Can you work these out from the model? Positions are in its coordinate system, mm. A direction names the side the tool comes from. Give positions to 0.01 mm unless a question says otherwise; leave off trailing zeros. Write each loop counter-clockwise with the first axis right and the second up, starting at its lowest first coordinate (ties: lowest second). Pieces come first, ordered by that corner, then holes. Notation, with made-up numbers: (28.25, 74.5) -> (44.25, 74.5) arc R28 ccw to (44.25, 93.5) -> close; hole circle Ø8 at (36.25, 29.25). An arc over 180 degrees is marked (long way). One line per item, written item: value.
from build123d import *

# Parameters (mm, degrees)
F0_W     = 65
F0_H     = 25
F1_DEPTH = 2
F2_W     = 3
F2_H     = 25
F3_DEPTH = 66
F4_R     = 4
F4_R_2   = 1.5
F5_DEPTH = 65.001


with BuildPart() as f1:
    # F0 (on Top) → F1 (new body)
    with BuildSketch(Plane.XY):
        with Locations((32.5, 12.5)):
            Rectangle(F0_W, F0_H)
    extrude(amount=F1_DEPTH)

    # F2 (on Top) → F3 (join)
    with BuildSketch(Plane.XY):
        with Locations((1.5, 12.5)):
            Rectangle(F2_W, F2_H)
        with Locations((63.5, 12.5)):
            Rectangle(F2_W, F2_H)
    extrude(amount=F3_DEPTH)

    # F4 (on face) → F5 (cut, through all)
    with BuildSketch(Plane(origin=(0, 0, 0), x_dir=(0, -1, 0), z_dir=(-1, 0, 0))):
        with BuildLine():
            ThreePointArc((-25, 53.5), (-21.338835, 62.338835), (-12.5, 66))
            Line((-12.5, 66), (-25, 66))
            Line((-25, 66), (-25, 53.5))
        make_face()
        with BuildLine():
            ThreePointArc((-12.5, 66), (-3.661165, 62.338835), (0, 53.5))
            Line((0, 53.5), (0, 66))
            Line((0, 66), (-12.5, 66))
        make_face()
        with Locations((-12.5, 53.5)):
            Circle(F4_R)
        with Locations((-12.5, 60.5)):
            Circle(F4_R_2)
        with Locations((-19.5, 53.5)):
            Circle(F4_R_2)
        with Locations((-12.5, 46.5)):
            Circle(F4_R_2)
        with Locations((-5.5, 53.5)):
            Circle(F4_R_2)
    extrude(amount=-F5_DEPTH, mode=Mode.SUBTRACT)


solid = f1.part
1) Will this pin go through, and if not, where does the flat tip stop? pin 1 (1.5 mm diameter, centred on x = 24.5, y = 5.5, fed in from +Z).
Answer list:
pin 1: stops at z = 2
2) If we section it at C-C (z = 60.5): Write out the boundary of the cut face in (x, y).
Answer list:
outline: (0, 2.14) -> (3, 2.14) -> (3, 11) -> (0, 11) -> close; (0, 14) -> (3, 14) -> (3, 22.86) -> (0, 22.86) -> close; (62, 2.14) -> (65, 2.14) -> (65, 11) -> (62, 11) -> close; (62, 14) -> (65, 14) -> (65, 22.86) -> (62, 22.86) -> close
3) I need wall thicknesses on L1, parallel to Z at x = 63.25, y = 12.5; L2, parallel to X at y = 20.75, z = 54.5; L3, parallel to Z at x = 0.9, y = 19.5. Which ranges of each line are inside material? Lowest first, please.
Answer list:
L1: z = 0 to 45, 48 to 49.5, 57.5 to 59, 62 to 66
L2: x = 0 to 3, 62 to 65
L3: z = 0 to 52, 55 to 63.86
4) If we section it at A-A (z = 9.5): Write out the boundary of the cut face in (x, y), and give its area (3 significant figures).
Answer list:
outline: (0, 0) -> (3, 0) -> (3, 25) -> (0, 25) -> close; (62, 0) -> (65, 0) -> (65, 25) -> (62, 25) -> close
area: 150 mm^2
5) We'd pull the mould along X, two halves only. Please class faces 3 (the face through (3, 12, 34)), 4 (the face through (65, 12, 33)), 5 (the face through (1.479, 12.695, 61.987)): released by +X, released by -X, zero draft, split by the parting line, or undercut.
Answer list:
face 3: undercut
face 4: released by +X
face 5: zero draft
6) For faces 1 (the face through (62, 12, 34)), 2 (the face through (1.479, 13.367, 49.595)), which set-ups out of +Z, -Z, +X, -X, +Y, -Y let a thin tool reach every point of the face, with its end or its side?
Answer list:
face 1: +Z, +Y, -Y
face 2: +X, -X
7) If we section it at D-D (y = 2): Write out the boundary of the cut face in (x, z).
Answer list:
outline: (0, 0) -> (65, 0) -> (65, 60.28) -> (62, 60.28) -> (62, 2) -> (3, 2) -> (3, 60.28) -> (0, 60.28) -> close
8) If we section it at B-B (y = 19.5): Write out the boundary of the cut face in (x, z), and give its area (3 significant figures).
Answer list:
outline: (0, 0) -> (65, 0) -> (65, 52) -> (62, 52) -> (62, 2) -> (3, 2) -> (3, 52) -> (0, 52) -> close; (0, 55) -> (3, 55) -> (3, 63.86) -> (0, 63.86) -> close; (62, 55) -> (65, 55) -> (65, 63.86) -> (62, 63.86) -> close
area: 483 mm^2
